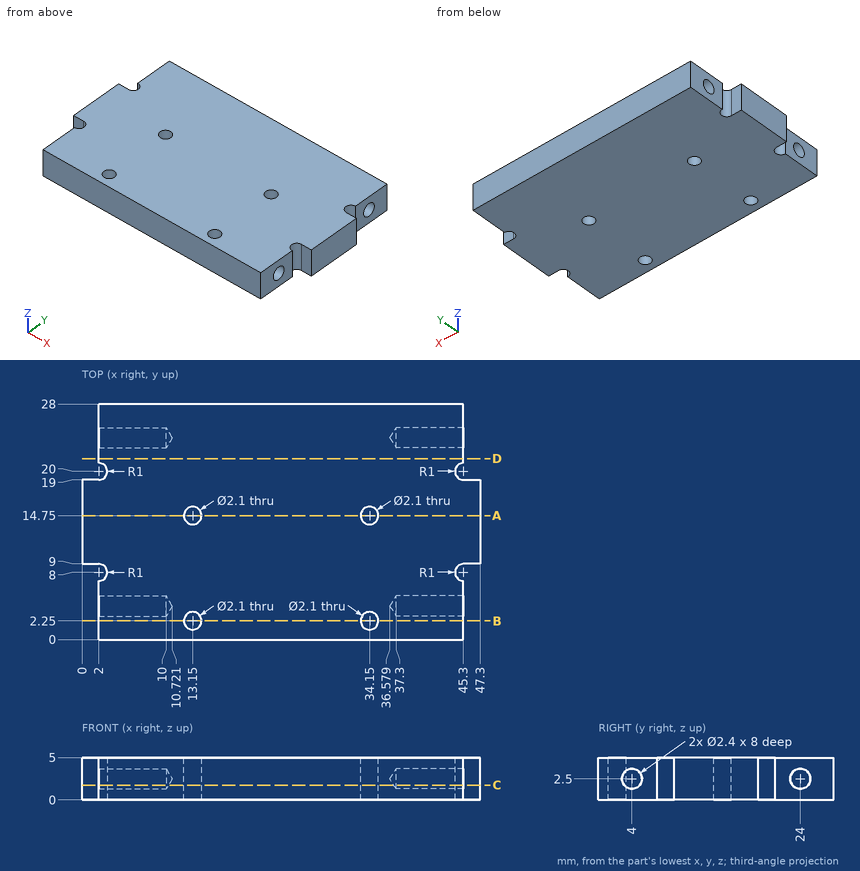
Answer from the drawing. Dimensions are ordinates in mm from the lowest x, y and z of the part. Coordinates: 2 decimals unless noted, no trailing zeros. Write each loop counter-clockwise with the first axis right and the second up, starting at its lowest first coordinate (ties: lowest second). Pieces come first, ordered by that corner, then holes. Notation, with made-up numbers: M 68,-27 L 80,-27 A9 ccw 80,-19 Z; hole C 62.5,59.5 d8. An arc over 180 degrees is marked long. Use one line per item in the form item = value. Start each with the question number.
1. Each of these flat-tipped pins is pushed along its axis until it touches: P1, Ø1.5, axis at y = 7, z = 2.5, coming from the +X side; P2, Ø1, axis at x = 46.5, z = 1.5, coming from the -Y side; P3, Ø3, axis at y = 24, z = 2.5, coming from the -X side. Where does it stop, or does it pass through?
2. Straight lines are drawn through the part: probe 1 along X at (y, z) = (14.75, 2.55); probe 2 along Y at (x, z) = (42.75, 2.5); probe 3 along X at (y, z) = (2.25, 2.3). For each, find the intervals that lie inside material, in ascending order. Write a range as from..to.
3. The part is cut by section D-D (y = 21.5). Give the vertices of the cut face in (x, z).
4. The part is cut by section C-C (z = 1.75). Give the number of separate pieces and of enclosed holes in the cut face, plus the area to 3 significant figures.
5. The part is cut by section A-A (y = 14.75). Give the vertices of the cut face in (x, z).
6. The part is cut by section B-B (y = 2.25). Give the vertices of the cut face in (x, z), plus the area to 4 significant figures.
Evaluation:
q1.P1 = 45.3
q1.P2 = 9
q1.P3 = 2
q2.probe_1 = 0..12.1, 14.2..33.1, 35.2..47.3
q2.probe_2 = 0..2.8, 5.2..22.8, 25.2..28
q2.probe_3 = 2..12.1, 14.2..33.1, 35.2..45.3
q3.outline = M 2,0 L 45.3,0 L 45.3,5 L 2,5 Z
q4.separate_pieces = 1
q4.enclosed_holes = 4
q4.area = 1,170 mm^2
q5.outline = M 0,0 L 12.1,0 L 12.1,5 L 0,5 Z; M 14.2,0 L 33.1,0 L 33.1,5 L 14.2,5 Z; M 35.2,0 L 47.3,0 L 47.3,5 L 35.2,5 Z
q6.outline = M 2,0 L 12.1,0 L 12.1,5 L 2,5 Z; M 14.2,0 L 33.1,0 L 33.1,5 L 14.2,5 Z; M 35.2,0 L 45.3,0 L 45.3,5 L 35.2,5 Z
q6.area = 195.5 mm^2
